Geometry: see drawing. Coordinates: mm, zero at the bounding-box minimum. A direction names the side the tool comes from. Coordinates: 2 decimals unless noted, no trailing zeros. Write each loop counter-clockwise with the first axis right and the second up, starting at its lowest first coordinate (ties: lowest second). Pieces come first, ordered by that corner, then holes. Notation, with made-up numbers: M 88.5,0 L 145.5,0 A19 ccw 145.5,24 Z; hole C 80.5,-37 d7. An arc over 180 degrees is marked long. Answer as CSV lines item,"result". Start each with the question number.
1. Reachability of the marked faces 4, 5 and 6 from +Z, -Z, +X, -X, +Y, -Y: full face, straight path, thin tool, end or side. Return the list, or none.
2. Line query: probe 1 along X at (y, z) = (69, 14); probe 2 along Z at (x, y) = (44, 71); probe 3 along X at (y, z) = (66, 19). Output: solid intervals per line, ascending. Write a range as [from, to].
3. Section C-C on x = 527.05. Return the cut outline in (y, z).
4. Contact query for flat-ended pins moving along their axis: pin 1 Ø4 at (x, z) = (174.5, 25) entering from -Y; pin 2 Ø8.5 at (x, z) = (44.45, 19.05) entering from -Y; pin 3 Ø3 at (y, z) = (43.5, 2.5) entering from -X; pin 4 Ø8 at (y, z) = (37.5, 29.5) entering from +X. Output: stop coordinate, or through.
5. Section A-A on z = 19.05. Count the separate pieces of the cut face and the enclosed holes in it, plus the area to 3 significant figures.
6. Mould query, pull axis Y, two halves, no side actions, for the marked faces 1, 2 and 3. Classes: pulls with the +Y half, pulls with the -Y half, needs draft (parallel to the pull), parting line crosses it, or undercut.
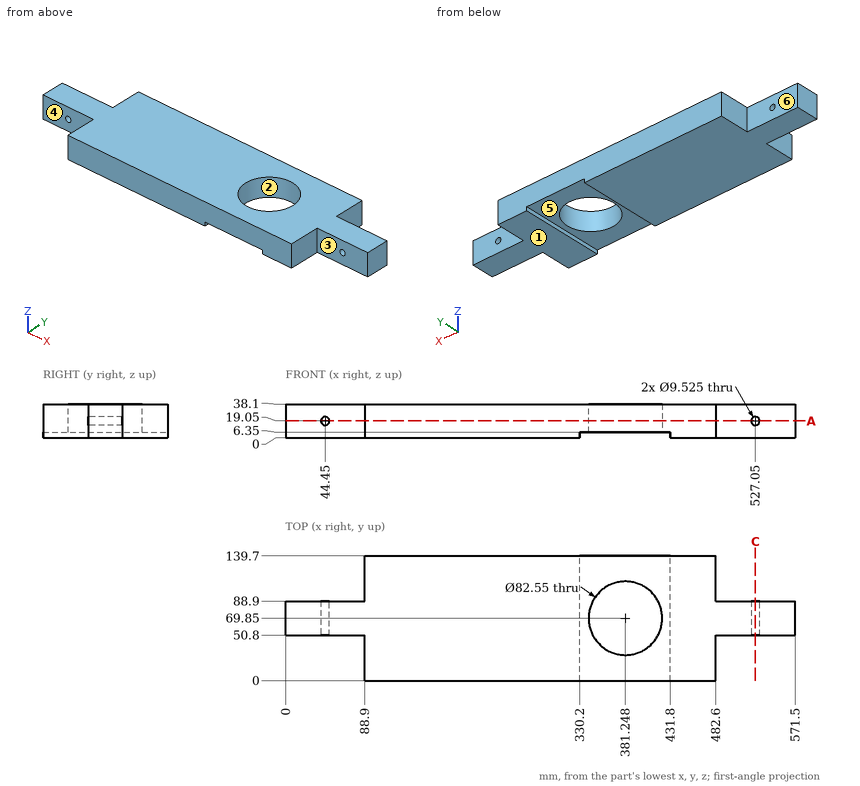
Values:
1,face 4,"+Z, -Z, -X, -Y"
1,face 5,"-Z, +Y, -Y"
1,face 6,"+Z, -Z, -X, +Y"
2,probe 1,"[0, 339.98], [422.51, 571.5]"
2,probe 2,"[0, 14.31], [23.79, 38.1]"
2,probe 3,"[0, 39.69], [49.21, 340.15], [422.34, 522.29], [531.81, 571.5]"
3,outline,"M 50.8,0 L 88.9,0 L 88.9,14.29 L 50.8,14.29 Z; M 50.8,23.81 L 88.9,23.81 L 88.9,38.1 L 50.8,38.1 Z"
4,pin 1,"y = 0"
4,pin 2,"through"
4,pin 3,"x = 88.9"
4,pin 4,"x = 482.6"
5,separate pieces,"3"
5,enclosed holes,"1"
5,area,"55,700 mm²"
6,face 1,"needs draft"
6,face 2,"undercut"
6,face 3,"pulls with the -Y half"
